Check sheet for the modelled part. Datum: model origin and axes. Units: mm. Face numbers are marked on the shaded views. A direction names the side the tool comes from. Coordinates: 2 decimals unless noted, no trailing zeros. Loops run counter-clockwise (first coordinate to the right, second up) from the corner with the lowest first, then second, coordinate; pieces in that order, holes last. Notation, with made-up numbers: (44.25, 52) - (54.25, 52) arc R12 cw to (54.25, 57) - close; hole circle Ø7 at (-21, 11). An arc over 180 degrees is marked (long way). Use a Markdown table: item, result. Add a question column.
1) Sectioned sample at B-B, the plane y = 24. Enter the section's corners in (x, z).
2) Thickness scan on line 1 (Y direction, x = -2.25, z = -3.5) (3 decimals); line 2 (X direction, y = 10.5, z = 1.75); line 3 (X direction, y = 22.5, z = 1). Record the ranges inside material, lowest first.
3) Tool access check on the marked faces 1, 2 and 3. Record the directions out of +Z, -Z, +X, -X, +Y, -Y that give a thin tool (end or side, any length) a straight path to the whole face; none if there is none.
4) Go/stop test with flat-tipped pins: P1, Ø6, axis at y = 11, z = -3, coming from the -X side; P2, Ø2, axis at y = 4.5, z = -2, coming from the -X side; P3, Ø1.6, axis at y = 29, z = 0, coming from the -X side. Record where each tip stops, or that it passes through.
from build123d import *

# Parameters (mm, degrees)
CUT_EXTRUDE1_DEPTH = 6.35
FILLET1_R          = 0.79375
FILLET2_R          = 0.79375
CHAMFER1_SIZE      = 0.254


with BuildPart() as part:
    # Sketch1 → Revolve1 (revolve)
    with BuildSketch(Plane.XY, mode=Mode.PRIVATE) as revolve1_sk:
        Polygon((0, 0), (5.55625, 0), (5.55625, 3.175), (2.38125, 3.175), (2.38125, 32.54375), (0, 32.54375), align=None)
    revolve(revolve1_sk.sketch.rotate(Axis((0, 3.469370861, 0), (0, -1, 0)), 90), axis=Axis((0, 3.469370861, 0), (0, -1, 0)))

    # Sketch4 → Cut-Extrude1 (cut)
    with BuildSketch(Plane(origin=(0, 32.54375, 0), x_dir=(1, 0, 0), z_dir=(0, 1, 0))):
        with BuildLine():
            Line((-2.270399729, -0.71807843), (-2.270399729, 0.71807843))
            ThreePointArc((-2.270399729, 0.71807843), (-2.38125, 0), (-2.270399729, -0.71807843))
        make_face()
        with BuildLine():
            Line((1.984375, -1.316285464), (1.984375, 1.316285464))
            ThreePointArc((1.984375, 1.316285464), (2.38125, 0), (1.984375, -1.316285464))
        make_face()
    extrude(amount=-CUT_EXTRUDE1_DEPTH, mode=Mode.SUBTRACT)

    # Fillet1
    fillet1_edges = [part.edges().sort_by_distance(p)[0] for p in [
        (0, 3.175, -2.38125),
    ]]
    fillet(fillet1_edges, radius=FILLET1_R)

    # Fillet2
    # the kernel refuses this fillet: 0.79375 mm, written as the material it adds along each edge
    with BuildSketch(Plane(origin=(1.984375, 26.19375, 3.300660464), x_dir=(0, 1, 0), z_dir=(0, 0, -1))) as fillet2_piece_1_section:
        with BuildLine():
            CenterArc((FILLET2_R, FILLET2_R), FILLET2_R, 180, 90)
            Line((0, FILLET2_R), (0, 0))
            Line((0, 0), (FILLET2_R, 0))
        make_face()
    fillet2_piece_1 = extrude(amount=6.601320927, mode=Mode.PRIVATE)
    fillet2_piece_1 = fillet2_piece_1 & Plane(origin=(0, 26.406315187, 0), x_dir=(0, 0, 1), z_dir=(0, 1, 0)) * Cylinder(2.38125, 17, mode=Mode.PRIVATE)
    add(fillet2_piece_1)
    with BuildSketch(Plane(origin=(-2.270399729, 26.19375, 2.70245343), x_dir=(0, 1, 0), z_dir=(0, 0, -1))) as fillet2_piece_2_section:
        with BuildLine():
            CenterArc((FILLET2_R, -FILLET2_R), FILLET2_R, 90, 90)
            Line((0, -FILLET2_R), (0, 0))
            Line((0, 0), (FILLET2_R, 0))
        make_face()
    fillet2_piece_2 = extrude(amount=5.404906861, mode=Mode.PRIVATE)
    fillet2_piece_2 = fillet2_piece_2 & Plane(origin=(0, 26.476974143, 0), x_dir=(0, 0, 1), z_dir=(0, 1, 0)) * Cylinder(2.38125, 14, mode=Mode.PRIVATE)
    add(fillet2_piece_2)

    # Chamfer1
    # the kernel refuses this chamfer: 0.254 mm, written as the material it takes off along each edge
    with BuildSketch(Plane(origin=(0, 32.54375, 0), x_dir=(-0.9994949156693064, 0, -0.03177913704312948), z_dir=(-0.03177913704312948, 0, 0.9994949156693064))) as chamfer1_piece_1:
        Polygon((2.38125, CHAMFER1_SIZE), (2.38125 - CHAMFER1_SIZE, 0), (2.38125, 0), align=None)
    revolve(axis=Axis((0, 32.54375, 0), (0, -1, 0)), revolution_arc=160.351494941, mode=Mode.SUBTRACT)
    with BuildSketch(Plane(origin=(0, 32.54375, 0), x_dir=(0, 0, 1), z_dir=(1, 0, 0))) as chamfer1_piece_2:
        Polygon((2.38125, CHAMFER1_SIZE), (2.38125 - CHAMFER1_SIZE, 0), (2.38125, 0), align=None)
    revolve(axis=Axis((0, 32.54375, 0), (0, -1, 0)), revolution_arc=88.170020766, mode=Mode.SUBTRACT)
    with BuildSketch(Plane(origin=(1.984375, 32.54375, 1.969492943), x_dir=(-0.9996219169112972, 0.027495876610573698, 0), z_dir=(0, 0, -1))) as chamfer1_piece_3:
        Polygon((CHAMFER1_SIZE * 0.999621916911, -CHAMFER1_SIZE * 0.0274958766106), (-CHAMFER1_SIZE * 0.0274958766106, -CHAMFER1_SIZE * 0.999621916911), (0, 0), align=None)
    extrude(amount=3.938985885, mode=Mode.SUBTRACT)
    with BuildSketch(Plane(origin=(-2.270399729, 32.54375, 1.371285909), x_dir=(-0.027495876610587867, -0.9996219169112968, 0), z_dir=(0, 0, -1))) as chamfer1_piece_4:
        Polygon((CHAMFER1_SIZE * 0.999621916911, -CHAMFER1_SIZE * 0.0274958766106), (-CHAMFER1_SIZE * 0.0274958766106, -CHAMFER1_SIZE * 0.999621916911), (0, 0), align=None)
    extrude(amount=2.742571819, mode=Mode.SUBTRACT)
    with BuildSketch(Plane(origin=(0, 3.175, 0), x_dir=(0, 0, 1), z_dir=(1, 0, 0))) as chamfer1_piece_5:
        Polygon((5.55625 - CHAMFER1_SIZE, 0), (5.55625, CHAMFER1_SIZE), (5.55625, 0), align=None)
    revolve(axis=Axis((0, 3.175, 0), (0, -1, 0)), mode=Mode.SUBTRACT)
    with BuildSketch(Plane(origin=(0, 0, 0), x_dir=(0, 0, 1), z_dir=(1, 0, 0))) as chamfer1_piece_6:
        Polygon((5.55625, -CHAMFER1_SIZE), (5.55625 - CHAMFER1_SIZE, 0), (5.55625, 0), align=None)
    revolve(axis=Axis((0, 0, 0), (0, -1, 0)), mode=Mode.SUBTRACT)
    with BuildSketch(Plane(origin=(0, 32.54375, 0), x_dir=(0.9519271960907222, 0, 0.3063243596954961), z_dir=(0.3063243596954961, 0, -0.9519271960907222))) as chamfer1_piece_7:
        Polygon((2.38125, CHAMFER1_SIZE), (2.38125 - CHAMFER1_SIZE, 0), (2.38125, 0), align=None)
    revolve(axis=Axis((0, 32.54375, 0), (0, -1, 0)), revolution_arc=72.162141692, mode=Mode.SUBTRACT)


solid = part.part
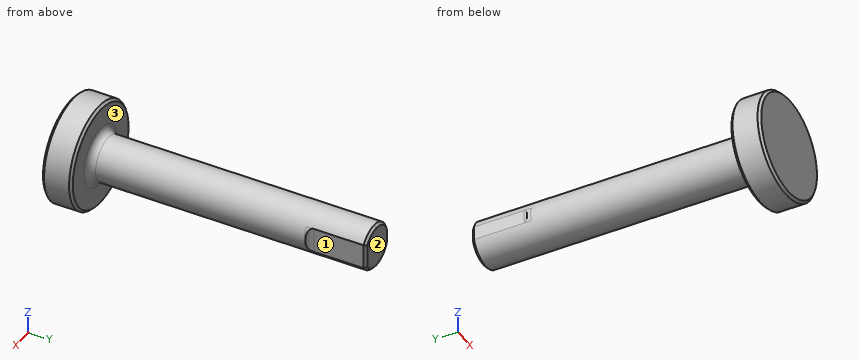
Solved:
| question | item | result |
|---|---|---|
| 1 | outline | circle Ø4.76 at (0, 0) |
| 2 | line 1 | y = 0 to 3.175 |
| 2 | line 2 | x = -1.61 to 1.61 |
| 2 | line 3 | x = -2.16 to 2.16 |
| 3 | face 1 | +Z, -Z, +X, +Y |
| 3 | face 2 | +Z, -Z, +X, -X, +Y |
| 3 | face 3 | +Y |
| 4 | P1 | stops at x = -2.38 |
| 4 | P2 | stops at x = -2.16 |
| 4 | P3 | stops at x = -2.27 |
